Read the model definition and answer for the solid it produces. Units are mm, in the model's axes. Face numbers are marked on the shaded views. Give positions to 0.01 mm unless a question says otherwise; leave off trailing zeros. Write each loop counter-clockwise with the first axis right and the second up, starting at its lowest first coordinate (ties: lowest second). Pieces come first, ordered by that corner, then holes. Notation, with made-up numbers: M 56,-28.75 L 103,-28.75 A22 ccw 103,6.25 Z; hole C 28.25,35 d6. An arc over 180 degrees is marked long. Put each result on its own line as item: value.
from build123d import *

# Parameters (mm, degrees)
SKETCH1_R               = 17
BOSS_EXTRUDE1_DEPTH     = 12
SKETCH2_R               = 17
SKETCH2_R_2             = 16
BOSS_EXTRUDE2_DEPTH     = 28
CUT_EXTRUDE1_DEPTH      = 47.669047558
CUT_EXTRUDE1_DEPTH_BACK = 47.669047558
SKETCH3_R               = 2.5
FILLET1_R               = 2


with BuildPart() as part:
    # Sketch1 → Boss-Extrude1 (new body)
    with BuildSketch(Plane.XY):
        Circle(SKETCH1_R)
    extrude(amount=BOSS_EXTRUDE1_DEPTH)

    # Sketch2 → Boss-Extrude2 (add)
    with BuildSketch(Plane.XY.offset(12)):
        Circle(SKETCH2_R)
        Circle(SKETCH2_R_2, mode=Mode.SUBTRACT)
    extrude(amount=BOSS_EXTRUDE2_DEPTH)

    # Sketch3 → Cut-Extrude1 (cut, two sides: drawn at the far end of the back side and taken through both)
    with BuildSketch(Plane(origin=(0, 0, 0), x_dir=(1, 0, 0), z_dir=(0, 1, 0)).offset(-CUT_EXTRUDE1_DEPTH_BACK)):
        with Locations(Location((0, -24, 0), (0, 0, 270))):
            Circle(SKETCH3_R)
    extrude(amount=CUT_EXTRUDE1_DEPTH + CUT_EXTRUDE1_DEPTH_BACK, mode=Mode.SUBTRACT)

    # Fillet1
    fillet1_edges = [part.edges().sort_by_distance(p)[0] for p in [
        (-17, 0, 0),
    ]]
    fillet(fillet1_edges, radius=FILLET1_R)


solid = part.part
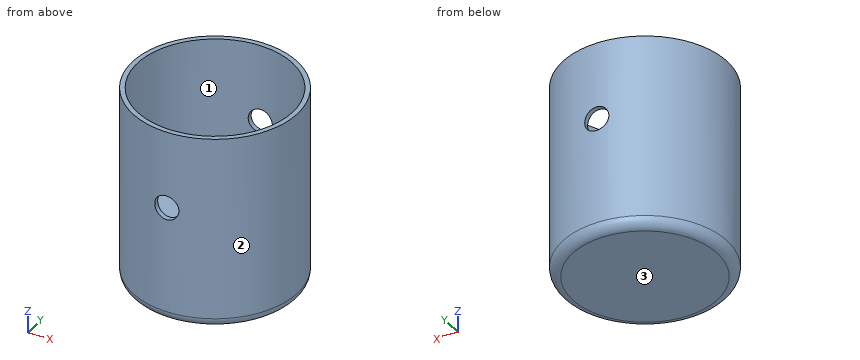
(1) Straight lines are drawn through the part: line 1 along Z through (x, y) = (13, 5); line 2 along Y through (x, z) = (0.5, 5); line 3 along X through (y, z) = (2.5, 26). For each, find the intervals that lie inside material, in ascending order. Write a range as from..to.
Result:
line 1: z = 0..12
line 2: y = -16.99..16.99
line 3: x = -16.82..-15.8, 15.8..16.82
(2) Section A-A on x = 0 is taken. Determine the outline of the cut face in (y, z).
Result:
outline: M -17,2 A2 ccw -15,0 L 15,0 A2 ccw 17,2 L 17,21.5 L 16,21.5 L 16,12 L -16,12 L -16,21.5 L -17,21.5 Z; M -17,26.5 L -16,26.5 L -16,40 L -17,40 Z; M 16,26.5 L 17,26.5 L 17,40 L 16,40 Z
(3) For a pull along Y with two mould halves and no side action, classify the marked faces 1, 2 and 3 as +Y half, -Y half, draft (parallel to the pull), parting line (faces both ways), or undercut.
Result:
face 1: undercut
face 2: parting line
face 3: draft
(4) Section C-C on y = 0 is taken. Determine the outline of the cut face in (x, z).
Result:
outline: M -17,2 A2 ccw -15,0 L 15,0 A2 ccw 17,2 L 17,40 L 16,40 L 16,12 L -16,12 L -16,40 L -17,40 Z
(5) Given pin 1 Ø4 at (y, z) = (-9, 29.5) entering from -X; pin 2 Ø5 at (x, z) = (9.5, 28.5) entering from +Y; pin 3 Ø5 at (y, z) = (3.5, 14.5) entering from -X, each flat-ended and moving along its own axis, determine where each tip first touches the part or whether it passes through.
Result:
pin 1: stops at x = -15.49
pin 2: stops at y = 15.49
pin 3: stops at x = -16.97
(6) Section D-D on z = 18 is taken. Determine the outline of the cut face in (x, y).
Result:
outline: C 0,0 d34; hole C 0,0 d32
